Here's how the part is built. I have some questions about the finished solid (model axes, mm). Give positions to 0.01 mm unless a question says otherwise; leave off trailing zeros. Write each loop counter-clockwise with the first axis right and the second up, starting at its lowest first coordinate (ties: lowest second). Pieces come first, ordered by that corner, then holes. Notation, with made-up numbers: (-25.5, 46) -> (31.5, 46) arc R13 cw to (31.5, 52) -> close; hole circle Ø2 at (38.25, 30). An arc over 180 degrees is marked (long way). Answer as CSV lines item,"result". Start each with the question number.
from build123d import *

# Parameters (mm, degrees)
SKETCH1_W           = 160
SKETCH1_H           = 35
BOSS_EXTRUDE1_DEPTH = 5
CHAMFER1_SIZE       = 10
SKETCH2_W           = 1
SKETCH2_H           = 15
BOSS_EXTRUDE2_DEPTH = 0.5


with BuildPart() as part:
    # Sketch1 → Boss-Extrude1 (new body)
    with BuildSketch(Plane(origin=(0, 0, 0), x_dir=(1, 0, 0), z_dir=(0, 1, 0))):
        Rectangle(SKETCH1_W, SKETCH1_H)
    extrude(amount=BOSS_EXTRUDE1_DEPTH)

    # Chamfer1
    # the kernel refuses this chamfer: 10 mm, written as the material it takes off along each edge
    with BuildSketch(Plane(origin=(105.71682988, 5, -17.5), x_dir=(0, -0.9996219169112968, -0.027495876610586317), z_dir=(-1, 0, 0)), Plane(origin=(-105.71682988, 5, 17.5), x_dir=(0, -0.9996219169112968, 0.027495876610586317), z_dir=(1, 0, 0))) as chamfer1_piece_1:
        Polygon((CHAMFER1_SIZE * 0.999621916911, CHAMFER1_SIZE * 0.0274958766106), (-CHAMFER1_SIZE * 0.0274958766106, CHAMFER1_SIZE * 0.999621916911), (0, 0), align=None)
    extrude(amount=211.433659759, mode=Mode.SUBTRACT)

    # Sketch2 → Boss-Extrude2 (add)
    with BuildSketch(Plane(origin=(0, 5, 0), x_dir=(1, 0, 0), z_dir=(0, 1, 0))):
        with Locations((72.5, 0)):
            Rectangle(SKETCH2_W, SKETCH2_H)
        with Locations((67.5, 0)):
            Rectangle(SKETCH2_W, SKETCH2_H)
        with Locations((62.5, 0)):
            Rectangle(SKETCH2_W, SKETCH2_H)
        with Locations((57.5, 0)):
            Rectangle(SKETCH2_W, SKETCH2_H)
        with Locations((52.5, 0)):
            Rectangle(SKETCH2_W, SKETCH2_H)
        with Locations((47.5, 0)):
            Rectangle(SKETCH2_W, SKETCH2_H)
        with Locations((42.5, 0)):
            Rectangle(SKETCH2_W, SKETCH2_H)
        with Locations((37.5, 0)):
            Rectangle(SKETCH2_W, SKETCH2_H)
        with Locations((32.5, 0)):
            Rectangle(SKETCH2_W, SKETCH2_H)
        with Locations((27.5, 0)):
            Rectangle(SKETCH2_W, SKETCH2_H)
        with Locations((22.5, 0)):
            Rectangle(SKETCH2_W, SKETCH2_H)
        with Locations((17.5, 0)):
            Rectangle(SKETCH2_W, SKETCH2_H)
        with Locations((12.5, 0)):
            Rectangle(SKETCH2_W, SKETCH2_H)
        with Locations((7.5, 0)):
            Rectangle(SKETCH2_W, SKETCH2_H)
        with Locations((2.5, 0)):
            Rectangle(SKETCH2_W, SKETCH2_H)
        with Locations((-2.5, 0)):
            Rectangle(SKETCH2_W, SKETCH2_H)
        with Locations((-7.5, 0)):
            Rectangle(SKETCH2_W, SKETCH2_H)
        with Locations((-12.5, 0)):
            Rectangle(SKETCH2_W, SKETCH2_H)
        with Locations((-17.5, 0)):
            Rectangle(SKETCH2_W, SKETCH2_H)
        with Locations((-22.5, 0)):
            Rectangle(SKETCH2_W, SKETCH2_H)
        with Locations((-27.5, 0)):
            Rectangle(SKETCH2_W, SKETCH2_H)
        with Locations((-32.5, 0)):
            Rectangle(SKETCH2_W, SKETCH2_H)
        with Locations((-37.5, 0)):
            Rectangle(SKETCH2_W, SKETCH2_H)
        with Locations((-42.5, 0)):
            Rectangle(SKETCH2_W, SKETCH2_H)
        with Locations((-47.5, 0)):
            Rectangle(SKETCH2_W, SKETCH2_H)
        with Locations((-52.5, 0)):
            Rectangle(SKETCH2_W, SKETCH2_H)
        with Locations((-57.5, 0)):
            Rectangle(SKETCH2_W, SKETCH2_H)
        with Locations((-62.5, 0)):
            Rectangle(SKETCH2_W, SKETCH2_H)
        with Locations((-67.5, 0)):
            Rectangle(SKETCH2_W, SKETCH2_H)
        with Locations((-72.5, 0)):
            Rectangle(SKETCH2_W, SKETCH2_H)
    extrude(amount=BOSS_EXTRUDE2_DEPTH)


solid = part.part
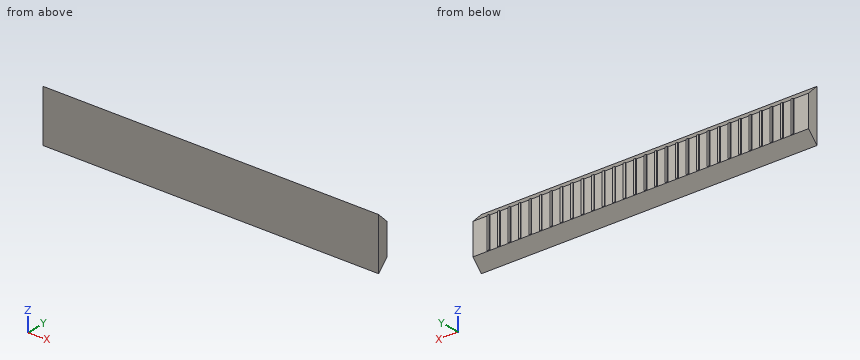
Item 1: If we section it at A-A (y = 2.75): Please give me the cut outline in (x, z), and give its area (3 significant figures).
Item 2: If I drill on line 1 (Y direction, x = -8, z = -9.5); line 2 (Y direction, x = -40, z = -4.5); line 3 (Z direction, x = 26, y = 4.3), over which ranges is the centre line in solid material (lowest first)? Write a range as [from, to].
Item 3: I'm going to push a flat-ended pin straight in: pin 1 (0.6 mm diameter, centred on x = -12.5, y = 5.5, fed in from +Z). Where does the tip first touch, or does it pass through?
Item 4: If we section it at B-B (x = -65.5): Please give me the cut outline in (y, z).
Final values:
1,outline,"(-80, -9.75) -> (80, -9.75) -> (80, 9.75) -> (-80, 9.75) -> close"
1,area,"3,120 mm2"
2,line 1,"[0, 3]"
2,line 2,"[0, 5]"
2,line 3,"[-8.2, 8.2]"
3,pin 1,"z = 7.5"
4,outline,"(0, -12.5) -> (5, -7.5) -> (5, 7.5) -> (0, 12.5) -> close"
